Source: CAD feature listing. Evaluate the final solid. Frame: model axes, mm. Coordinates: 2 decimals unless noted, no trailing zeros. Write each loop counter-clockwise with the first axis right and the second up, starting at its lowest first coordinate (ties: lowest second). Pieces come first, ordered by that corner, then holes. Notation, with made-up numbers: (18.25, -26.5) - (27.25, -26.5) arc R21 ccw to (27.25, -20.5) - close; hole circle Ø10 at (16, 52). An arc over 180 degrees is marked (long way). One line per question, with ' | ' between items.
Autodesk Inventor part; units mm, degrees
ref_plane "YZ Plane" through (0, 0, 0) normal (1, 0, 0) x (0, 1, 0)
ref_plane "XZ Plane" through (0, 0, 0) normal (0, 1, 0) x (-1, 0, 0)
ref_plane "XY Plane" through (0, 0, 0) normal (0, 0, 1) x (1, 0, 0)
sketch "Sketch1" plane through (0, 0, 0) normal (0, 0, 1) x (1, 0, 0)
  line L0 (0, 25.4) -> (0, 0)
  line L1 (0, 0) -> (25.4, 0)
  line L2 (3.175, 25.4) -> (3.175, 4.953)
  line L3 (4.953, 3.175) -> (25.4, 3.175)
  line L4 (0, 25.4) -> (3.175, 25.4)
  line L5 (25.4, 3.175) -> (25.4, 0)
  line L6 (3.175, 4.953) -> (3.175, 3.175)
  line L7 (4.953, 3.175) -> (3.175, 3.175)
  dimension "d0" = 25.4
  dimension "d1" = 25.4
  dimension "d2" = 3.175
extrude "Extrusion1" add sketch "Sketch1" along normal blind 492.125
sketch "Sketch2" plane through (3.175, 3.175, 0) normal (0, 1, 0) x (1, 0, 0)
  circle A0 centre (9.525, -479.425) radius 2.8398
  line L0 (22.225, -492.125) -> (0, -492.125)
  line L1 (22.225, 0) -> (22.225, -492.125)
  circle A1 centre (9.525, -12.7) radius 2.8398
  line L2 (22.225, 0) -> (0, 0)
  point P0 (-3.175, 0)
  point P1 (1.778, -492.125)
  point P2 (1.778, 0)
  dimension "d5" = 12.7
  dimension "d6" = 12.7
  dimension "d9" = 466.725
  dimension "d31" = 12.7
hole "Hole1" at (12.7, 3.175, 479.425) at (12.7, 3.175, 12.7) direction (0, -1, 0) diameter 6.7564 depth 25.4 tip angle 118
sketch "Sketch8" plane through (3.175, 3.175, 0) normal (0, 1, 0) x (1, 0, 0)
  circle A0 centre (9.525, -451.485) radius 5.9545
  line L0 (22.225, 0) -> (22.225, -492.125)
  line L1 (22.225, -492.125) -> (0, -492.125)
  point P0 (-3.175, 0)
  dimension "d59" = 12.7
  dimension "d60" = 40.64
hole "Hole5" at (12.7, 3.175, 451.485) direction (0, -1, 0) diameter 6.7564 depth 25.4 tip angle 118
sketch "Sketch9" plane through (3.175, 3.175, 0) normal (0, 1, 0) x (1, 0, 0)
  circle A0 centre (9.525, -40.64) radius 2.391
  line L0 (22.225, 0) -> (22.225, -492.125)
  line L1 (22.225, 0) -> (0, 0)
  point P0 (-3.175, 0)
  dimension "d68" = 12.7
  dimension "d69" = 40.64
hole "Hole6" at (12.7, 3.175, 40.64) direction (0, -1, 0) diameter 6.7564 depth 25.4 tip angle 118
sketch "Sketch10" plane through (3.175, 3.175, 0) normal (0, 1, 0) x (1, 0, 0)
  circle A0 centre (9.525, -134.62) radius 3.9264
  line L0 (22.225, 0) -> (22.225, -492.125)
  line L1 (22.225, 0) -> (0, 0)
  circle A1 centre (9.525, -246.38) radius 3.9264
  circle A2 centre (9.525, -358.14) radius 3.9264
  point P0 (-3.175, 0)
  dimension "d77" = 12.7
  dimension "d78" = 134.62
  dimension "d81" = 111.76
hole "Hole7" at (12.7, 3.175, 134.62) at (12.7, 3.175, 246.38) at (12.7, 3.175, 358.14) direction (0, -1, 0) diameter 6.7564 depth 25.4 tip angle 118
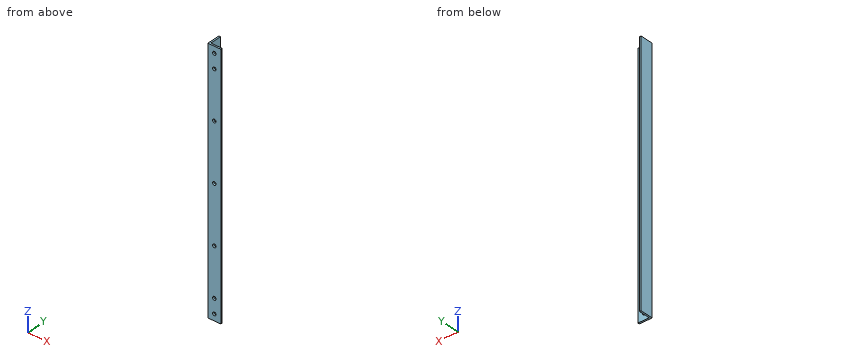
Item 1: Pin query (flat end, axial travel): pin 1 Ø8 at (x, z) = (12.7, 40.64) entering from +Y (3 decimals); pin 2 Ø4 at (y, z) = (21.5, 418) entering from +X (3 decimals); pin 3 Ø10 at (x, y) = (11, 20) entering from -Z. Return the tip coordinate at first contact, or that it passes through.
Check sheet entries:
pin 1: y = 3.175 | pin 2: x = 3.175 | pin 3: through
Item 2: Ray query, line 1 along X through (y, z) = (1.05, 134.62); line 2 along Y through (x, z) = (6, 215) (3 decimals). Return the intervals inside material, ascending. Write a range as [from, to].
Check sheet entries:
line 1: [0, 9.32], [16.08, 25.4] | line 2: [0, 3.175]
Item 3: Cut plane A-A on z = 69.5. Return loops of the section in (x, y) (3 decimals).
Check sheet entries:
outline: (0, 0) - (25.4, 0) - (25.4, 3.175) - (3.175, 3.175) - (3.175, 25.4) - (0, 25.4) - close
Item 4: Cut plane B-B on y = 16. Return loops of the section in (x, z) (3 decimals), and give its area (3 significant figures).
Check sheet entries:
outline: (0, 0) - (3.175, 0) - (3.175, 492.125) - (0, 492.125) - close | area: 1,560 mm²
